The listing builds one solid part. Answer for the finished solid, in the listing's coordinates (mm). A direction names the side the tool comes from. Round coordinates to 2 decimals unless told otherwise and drop trailing zeros. Loops run counter-clockwise (first coordinate to the right, second up) from the corner with the lowest first, then second, coordinate; pieces in that order, holes last. Notation, with made-up numbers: M 45,25.5 L 66,25.5 A28 ccw 66,60.5 Z; hole C 15,60.5 d2. An arc over 180 degrees is marked long. Answer as a JSON object with one key per item and string values.
```python
from build123d import *

# Parameters (mm, degrees)
F0_W     = 25.4
F0_H     = 19.05
F1_DEPTH = 19.05


with BuildPart() as f1:
    # F0 (on Front) → F1 (new body)
    with BuildSketch(Plane.XZ):
        with BuildLine():
            ThreePointArc((-16.695471328, 9.1740796342), (-4.7357032847, -18.4519813137), (19.05, 0))
            ThreePointArc((19.05, 0), (18.4519813137, 4.7357032847), (16.695471328, 9.1740796342))
            Line((16.695471328, 9.1740796342), (0, 9.1740796342))
            Line((0, 9.1740796342), (-16.695471328, 9.1740796342))
        make_face()
        with BuildLine():
            ThreePointArc((4.7625, 0), (-3.3675960454, -3.3675960454), (0, 4.7625))
            ThreePointArc((0, 4.7625), (3.3675960454, 3.3675960454), (4.7625, 0))
        make_face(mode=Mode.SUBTRACT)
        with BuildLine():
            Line((0, 9.1740796342), (16.695471328, 9.1740796342))
            ThreePointArc((16.695471328, 9.1740796342), (9.6988732069, 16.3961690195), (0, 19.05))
            Line((0, 19.05), (0, 9.1740796342))
        make_face()
        with BuildLine():
            ThreePointArc((0, 19.05), (9.6988732069, 16.3961690195), (16.695471328, 9.1740796342))
            Line((16.695471328, 9.1740796342), (55.88, 9.1740796342))
            Line((55.88, 9.1740796342), (55.88, 28.2240796342))
            Line((55.88, 28.2240796342), (36.83, 28.2240796342))
            Line((36.83, 28.2240796342), (11.43, 28.2240796342))
            Line((11.43, 28.2240796342), (-11.43, 28.2240796342))
            Line((-11.43, 28.2240796342), (-36.83, 28.2240796342))
            Line((-36.83, 28.2240796342), (-55.88, 28.2240796342))
            Line((-55.88, 28.2240796342), (-55.88, 9.1740796342))
            Line((-55.88, 9.1740796342), (-16.695471328, 9.1740796342))
            ThreePointArc((-16.695471328, 9.1740796342), (-9.6988732069, 16.3961690195), (0, 19.05))
        make_face()
        with BuildLine():
            ThreePointArc((0, 19.05), (-9.6988732069, 16.3961690195), (-16.695471328, 9.1740796342))
            Line((-16.695471328, 9.1740796342), (0, 9.1740796342))
            Line((0, 9.1740796342), (0, 19.05))
        make_face()
        with Locations((24.13, 37.7490796342)):
            Rectangle(F0_W, F0_H)
        with Locations((-24.13, 37.7490796342)):
            Rectangle(F0_W, F0_H)
    extrude(amount=F1_DEPTH)


solid = f1.part
```
Item 1: The part is cut by section D-D (x = 26.5). Give the vertices of the cut face in (y, z), then the cut area to 3 significant figures.
Values follow:
{"outline": "M -19.05,9.17 L 0,9.17 L 0,47.27 L -19.05,47.27 Z", "area": "726 mm^2"}
Item 2: Determine the mould class of faces 4 (the face through (11.43, -9, 38)), 5 (the face through (-36.83, -9, 38)), 6 (the face through (-1, -19.05, 22)), 7 (the face through (36.83, -9, 38)) for opening direction X: released by +X, released by -X, zero draft, split by the parting line, or undercut.
Values follow:
{"face 4": "undercut", "face 5": "released by -X", "face 6": "zero draft", "face 7": "released by +X"}
Item 3: The part is cut by section C-C (z = 3.5). Give the vertices of the cut face in (x, y), then the cut area to 3 significant figures.
Values follow:
{"outline": "M -18.73,-19.05 L -3.23,-19.05 L -3.23,0 L -18.73,0 Z; M 3.23,-19.05 L 18.73,-19.05 L 18.73,0 L 3.23,0 Z", "area": "590 mm^2"}
Item 4: Flat-ended cylindrical pins translate along their axes: P1, Ø10, axis at y = -6.5, z = -12.5, coming from the -X side; P2, Ø5.5, axis at y = -6.5, z = 39, coming from the -X side; P3, Ø5.5, axis at y = -9.5, z = 38.5, coming from the +X side; P4, Ø8.5, axis at x = 0, z = 0, coming from the -Y side. Find the tip coordinate at first contact, or state that the pin passes through.
Values follow:
{"P1": "x = -17.51", "P2": "x = -36.83", "P3": "x = 36.83", "P4": "through"}
Item 5: Which of the six approach directions +Z, -Z, +X, -X, +Y, -Y give full straight-line access (tool end or side, diameter ignored) to faces 1 (the face through (-46, -9, 28.224)), 2 (the face through (46, -9, 28.224)), 3 (the face through (0, -9, 28.224))?
Values follow:
{"face 1": "+Z, -X, +Y, -Y", "face 2": "+Z, +X, +Y, -Y", "face 3": "+Z, +Y, -Y"}
Item 6: The part is cut by section B-B (x = 0). Give the vertices of the cut face in (y, z), then the cut area to 3 significant figures.
Values follow:
{"outline": "M -19.05,-19.05 L 0,-19.05 L 0,-4.76 L -19.05,-4.76 Z; M -19.05,4.76 L 0,4.76 L 0,28.22 L -19.05,28.22 Z", "area": "719 mm^2"}
Item 7: Straight lines are drawn through the part: line 1 (X direction, y = -6.75, z = 0); line 2 (X direction, y = -14, z = 38); line 3 (Z direction, x = -17, y = -3.75). For each, find the intervals that lie inside material, in ascending order.
Values follow:
{"line 1": "-19.05 to -4.76, 4.76 to 19.05", "line 2": "-36.83 to -11.43, 11.43 to 36.83", "line 3": "-8.6 to 8.6, 9.17 to 47.27"}
